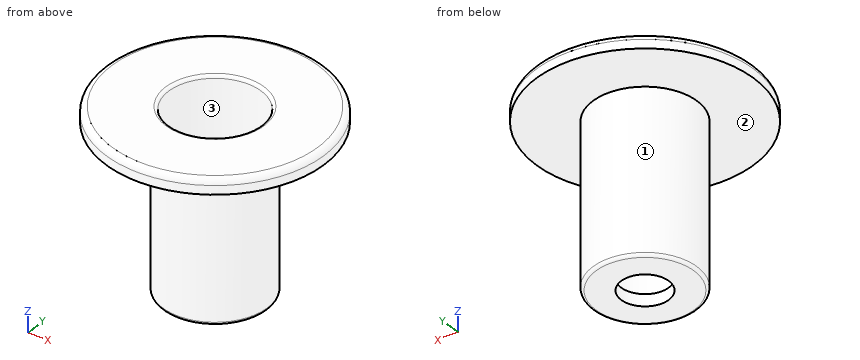
Solid Edge part; units mm, degrees
sketch "Sketch1" plane through (0, 0, 0) normal (0, 0, -1) x (-1, 0, 0)
  circle A0 centre (0, 0) radius 18.5
  circle A1 centre (0, 0) radius 7.85
extrude "Protrusion1" add sketch "Sketch1" along normal blind 2.5
sketch "Sketch2" plane through (0, 0, -2.5) normal (0, 0, -1) x (1, 0, 0)
  circle A0 centre (0, 0) radius 7.85
  circle A1 centre (0, 0) radius 8.85
extrude "Kihúzás_2" add sketch "Sketch2" along normal blind 27.5
sketch "Sketch3" plane through (0, 0, -30) normal (0, 0, -1) x (1, 0, 0)
  circle A0 centre (0, 0) radius 7.85
  circle A1 centre (0, 0) radius 4.05
extrude "Kihúzás_3" add sketch "Sketch3" against normal blind 2
fillet "Lekerekítés_2" radius 1 1 edges at (18.5, 0, 0)
fillet "Lekerekítés_3" radius 0.5 1 edges at (-8.85, 0, -30)
fillet "Lekerekítés_4" radius 0.5 1 edges at (7.85, 0, 0)
properties material "Polipropilén, általános rendeltetésű"
Verification items for the finished model (mm, model axes). Face numbers are marked on the shaded views. Round coordinates to 2 decimals unless told otherwise and drop trailing zeros. Loops run counter-clockwise (first coordinate to the right, second up) from the corner with the lowest first, then second, coordinate; pieces in that order, holes last. Notation, with made-up numbers: (-20, -23.5) - (27, -23.5) arc R17 ccw to (27, -17.5) - close; hole circle Ø1 at (-40, -11.5). An arc over 180 degrees is marked (long way). Write item = value, one per line.
Q1. Mould release check, pull along Y, two halves, no side actions. Record for the marked faces 1, 2 and 3: +Y half, -Y half, draft (parallel to the pull), parting line (faces both ways), or undercut.
Here are the results:
face_1 = parting line
face_2 = draft
face_3 = undercut
Q2. Sectioned sample at A-A on z = -18.75. Record the boundary of the cut face in (x, y).
Here are the results:
outline = circle Ø17.7 at (0, 0); hole circle Ø15.7 at (0, 0)
Q3. Material ranges on L1, parallel to X at y = 0, z = -28.55; L2, parallel to Y at x = 0, z = -11.25, recorded low to high.
Here are the results:
L1 = -8.85 to -4.05, 4.05 to 8.85
L2 = -8.85 to -7.85, 7.85 to 8.85
Q4. Depth check by flat-ended pin: pin 1 (5 mm diameter, centred on x = 0, y = 0, fed in from -Z); pin 2 (4 mm diameter, centred on x = -14, y = 14, fed in from +Z); pin 3 (6 mm diameter, centred on y = -8.5, z = -24, fed in from -X); pin 4 (4 mm diameter, centred on x = 3, z = -16, fed in from +Y). Enter the tip coordinate at first touch or a pass-through.
Here are the results:
pin_1 = through
pin_2 = -0.05
pin_3 = -6.93
pin_4 = 8.79
